```python
from build123d import *

# Parameters (mm, degrees)
EXTRUDE_1_DEPTH      = 33
EXTRUDE_1_DEPTH_BACK = 10
SKETCH_3_R           = 21.25
SKETCH_3_R_2         = 11.25
SKETCH_4_R           = 72.26496
EXTRUDE_1_2_DEPTH    = 27
SKETCH_2_R           = 15
CUT_EXTRUDE_1_DEPTH  = 220


with BuildPart() as part:
    # 草圖1 → 旋轉1 (revolve)
    with BuildSketch(Plane.XY, mode=Mode.PRIVATE) as revolve_1_sk:
        with BuildLine():
            Line((0, 0), (0, 70.143356265))
            Line((0, 70.143356265), (20, 70.143356265))
            Line((20, 70.143356265), (40, 50.650757283))
            add(Edge.make_bspline(
                [(40, 50.650757283), (85.38972146, 50.733312628), (143.705322116, 100.003369352), (176.495570272, 42.029481433)],
                knots=[0, 0, 0, 0, 1, 1, 1, 1], degree=3))
            Line((176.495570272, 42.029481433), (176.495570272, 0))
            Line((176.495570272, 0), (0, 0))
        make_face()
    revolve(revolve_1_sk.sketch.rotate(Axis((0, 0, 0), (1, 0, 0)), 90), axis=Axis((0, 0, 0), (1, 0, 0)))

    # 草圖3 → Extrude 1 (add, two sides: drawn at the far end of the back side and taken through both)
    with BuildSketch(Plane(origin=(0, -70, 0), x_dir=(1, 0, 0), z_dir=(0, 1, 0)).offset(-EXTRUDE_1_DEPTH_BACK)):
        with Locations((121.401340983, 0)):
            Circle(SKETCH_3_R)
        with Locations((121.401340983, 0)):
            Circle(SKETCH_3_R_2, mode=Mode.SUBTRACT)
    extrude(amount=EXTRUDE_1_DEPTH + EXTRUDE_1_DEPTH_BACK)

    # 草圖4 → Extrude 1 2 (add)
    with BuildSketch(Plane.ZY):
        Circle(SKETCH_4_R)
    extrude(amount=EXTRUDE_1_2_DEPTH)

    # 草圖2 → 除料-伸長1 (cut)
    with BuildSketch(Plane(origin=(176.495570272, 0, 0), x_dir=(0, 0, -1), z_dir=(1, 0, 0))):
        Circle(SKETCH_2_R)
    extrude(amount=-CUT_EXTRUDE_1_DEPTH, mode=Mode.SUBTRACT)


solid = part.part
```
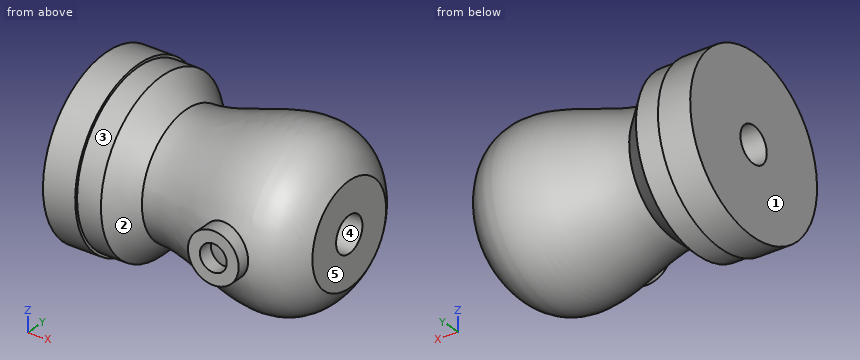
Read the model definition and answer for the solid it produces. Units are mm, in the model's axes. Face numbers are marked on the shaded views. A direction names the side the tool comes from. Give positions to 0.01 mm unless a question says otherwise; leave off trailing zeros. Write each loop counter-clockwise with the first axis right and the second up, starting at its lowest first coordinate (ties: lowest second). Pieces come first, ordered by that corner, then holes. Notation, with made-up numbers: M 34,24.25 L 55,24.25 A26 cw 55,47.25 Z; hole C -3.75,75 d3. An arc over 180 degrees is marked long. Put each result on its own line as item: value. Start each with the question number.
1. For a pull along Z with two mould halves and no side action, classify the marked faces 3, 4 and 5 as released by +Z, released by -Z, zero draft, split by the parting line, or undercut.
2. Consider line 1 along X through (y, z) = (-73, 0); line 2 along Z through (x, y) = (9, 7); line 3 along Y through (x, z) = (87, 3). Determine where each line is inside the solid, lowest interval first.
3. Which of the six approach directions +Z, -Z, +X, -X, +Y, -Y give full straight-line access (tool end or side, diameter ignored) to the marked faces 1 and 2?
4. The part is cut by section A-A, the plane x = -3. Give the vertices of the cut face in (y, z), and give its area (3 significant figures).
5. Each of these flat-tipped pins is pushed along its axis until it touches: pin 1 Ø13.5 at (x, z) = (121.4, 0) entering from -Y; pin 2 Ø3 at (x, z) = (53, 45.5) entering from -Y; pin 3 Ø3 at (x, y) = (85.5, 22.5) entering from -Z. Where does it stop, or does it pass through?
Final values:
1. face 3: split by the parting line
1. face 4: undercut
1. face 5: zero draft
2. line 1: x = 100.15 to 110.15, 132.65 to 142.65
2. line 2: z = -69.79 to -13.27, 13.27 to 69.79
2. line 3: y = -60.86 to -14.7, 14.7 to 60.86
3. face 1: +Z, -Z, -X, +Y, -Y
3. face 2: none
4. outline: C 0,0 d144.53; hole C 0,0 d30
4. area: 15,700 mm²
5. pin 1: stops at y = -70.18
5. pin 2: stops at y = -27.44
5. pin 3: stops at z = -56.9
